Input: part model. Units: mm. Frame: model coordinates. Face numbers are marked on the shaded views. Give positions to 0.01 mm unless a question says otherwise; leave off trailing zeros. Loops run counter-clockwise (first coordinate to the right, second up) from the corner with the lowest first, then second, coordinate; pieces in that order, holes last. Notation, with made-up numbers: (-0.75, 43.5) - (31.25, 43.5) arc R15 ccw to (31.25, 63.5) - close; hole circle Ø9 at (83, 43.25). An arc over 180 degrees is marked (long way). One line per item, written item: value.
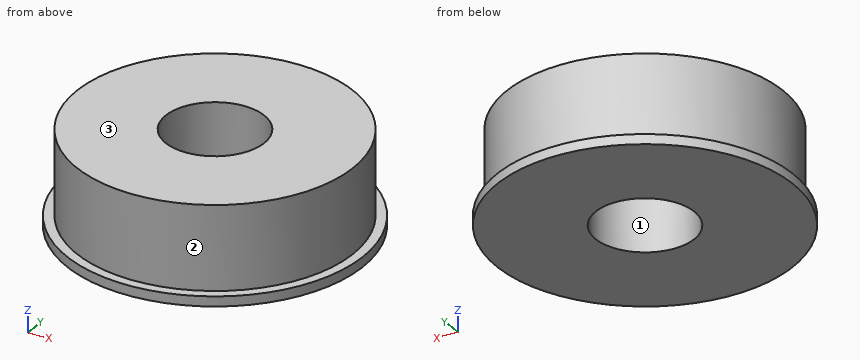
from build123d import *

# Parameters (mm, degrees)
F0_R     = 15
F1_DEPTH = 1
F2_R     = 14
F3_DEPTH = 8.5
F4_R     = 5
F5_DEPTH = 9.5


with BuildPart() as f1:
    # F0 (on Top) → F1 (new body)
    with BuildSketch(Plane.XY):
        Circle(F0_R)
    extrude(amount=F1_DEPTH)

    # F2 (on face) → F3 (join)
    with BuildSketch(Plane.XY.offset(1)):
        Circle(F2_R)
    extrude(amount=F3_DEPTH)

    # F4 (on face) → F5 (cut, through all)
    with BuildSketch(Plane.XY.offset(9.5)):
        Circle(F4_R)
    extrude(amount=-F5_DEPTH, mode=Mode.SUBTRACT)


solid = f1.part
Item 1: Section C-C, the plane z = 6.75. Output: boundary loops of the cut face in (x, y).
Verdict:
outline: circle Ø28 at (0, 0); hole circle Ø10 at (0, 0)
Item 2: Material intervals for L1, parallel to Y at x = 0, z = 6.5; L2, parallel to Z at x = -6, y = 13.25; L3, parallel to Y at x = 4.5, z = 7, sorted ascending.
Verdict:
L1: y = -14 to -5, 5 to 14
L2: z = 0 to 1
L3: y = -13.26 to -2.18, 2.18 to 13.26
Item 3: Pin query (flat end, axial travel): P1, Ø1.5, axis at y = -6, z = 8, coming from the +X side; P2, Ø1, axis at y = 7.5, z = 3, coming from the -X side. Return the tip coordinate at first contact, or that it passes through.
Verdict:
P1: stops at x = 12.98
P2: stops at x = -12.12
Item 4: Draft query along X for the marked faces 1, 2 and 3. Return one class per face: pulls with the +X half, pulls with the -X half, needs draft (parallel to the pull), parting line crosses it, or undercut.
Verdict:
face 1: undercut
face 2: parting line crosses it
face 3: needs draft
Item 5: Section A-A, the plane x = 0. Output: boundary loops of the cut face in (y, z), and give its area (3 significant figures).
Verdict:
outline: (-15, 0) - (-5, 0) - (-5, 9.5) - (-14, 9.5) - (-14, 1) - (-15, 1) - close; (5, 0) - (15, 0) - (15, 1) - (14, 1) - (14, 9.5) - (5, 9.5) - close
area: 173 mm^2
Item 6: Section D-D, the plane y = 9.5. Output: boundary loops of the cut face in (x, z).
Verdict:
outline: (-11.61, 0) - (11.61, 0) - (11.61, 1) - (10.28, 1) - (10.28, 9.5) - (-10.28, 9.5) - (-10.28, 1) - (-11.61, 1) - close
